from build123d import *

# Parameters (mm, degrees)
F0_W     = 30
F0_H     = 35
F0_H_2   = 5
F1_DEPTH = 4
F2_W     = 4.5
F2_H     = 40
F3_DEPTH = 7
F4_W     = 4.5
F4_H     = 40
F4_W_2   = 25.5
F5_DEPTH = 10
F7_D     = 6
F8_R     = 3
F9_DEPTH = 4.5
F10_SIZE = 8


# Not quite as in the source:
# - a feature names something its author has since deleted; it is built from what else it names


with BuildPart() as f1:
    # F0 (on Top) → F1 (new body)
    with BuildSketch(Plane.XY):
        with Locations((0, -22.5)):
            Rectangle(F0_W, F0_H)
        with Locations((0, -2.5)):
            Rectangle(F0_W, F0_H_2)
    extrude(amount=F1_DEPTH)

    # F2 (on face) → F3 (join)
    with BuildSketch(Plane.XY.offset(4)):
        with Locations((12.75, -20)):
            Rectangle(F2_W, F2_H)
        with Locations((-12.75, -20)):
            Rectangle(F2_W, F2_H)
    extrude(amount=F3_DEPTH)

    # F4 (on face) → F5 (join)
    with BuildSketch(Plane.XY.offset(11)):
        with Locations((12.75, -20)):
            Rectangle(F4_W, F4_H)
        with Locations((-2.25, -20)):
            Rectangle(F4_W_2, F4_H)
    extrude(amount=F5_DEPTH)

    # F7 (through all)
    with Locations(Plane.XY.offset(21)):
        with Locations((0, -20)):
            Hole(F7_D / 2)

    # F8 (on face) → F9 (cut)
    with BuildSketch(Plane(origin=(0, 0, 11), x_dir=(1, 0, 0), z_dir=(0, 0, -1))):
        Polygon((2.5980762114, 24.5), (-2.5980762114, 24.5), (-5.1961524227, 20), (-2.5980762114, 15.5), (2.5980762114, 15.5), (5.1961524227, 20), align=None)
        with Locations((0, 20)):
            Circle(F8_R, mode=Mode.SUBTRACT)
    extrude(amount=-F9_DEPTH, mode=Mode.SUBTRACT)

    # F10
    f10_edges = [f1.edges().sort_by_distance(p)[0] for p in [
        (-15, -20, 21),
        (15, -20, 21),
    ]]
    chamfer(f10_edges, length=F10_SIZE)


solid = f1.part
The model under review builds one solid part; all positions refer to its coordinate system, in mm. A direction names the side the tool comes from. Give positions to 0.01 mm unless a question says otherwise; leave off trailing zeros. Loops run counter-clockwise (first coordinate to the right, second up) from the corner with the lowest first, then second, coordinate; pieces in that order, holes last. Notation, with made-up numbers: (86.5, 58.25) -> (127.5, 58.25) arc R9 cw to (127.5, 64.25) -> close; hole circle Ø10 at (22, 62). An arc over 180 degrees is marked (long way). Answer as a JSON object with one key per item and string values. Group by question number.
Q1. Draft analysis for pull direction Z (two halves, no side actions). For faces 1 (the flat face through (0, -15.5, 13)), 2 (the flat face through (-4, -20, 0)), 3 (the flat face through (0, -40, 13)), state which applies: pulls with the +Z half, pulls with the -Z half, needs draft (parallel to the pull), parting line crosses it, or undercut.
Q2. Take a section at C-C (z = 12.25). Write out the cut boundary in (x, y).
Q3. Wall thickness on line 1 along Z through (x, y) = (-6.5, -22); line 2 along X through (y, z) = (-33, 9); line 3 along Y through (x, z) = (0, 16.95): over which ranges is each line inside the solid? List them lowest first.
Q4. Take a section at D-D (y = -16.5). Write out the cut boundary in (x, z), plus the area to 3 significant figures.
Q5. Take a section at A-A (x = 0). Write out the cut boundary in (y, z).
Q6. Insertion check: pin 1 (6 mm diameter, centred on x = 11, y = -10, fed in from +Z); pin 2 (2 mm diameter, centred on y = -31, z = 16, fed in from +X). Each pin has a flat end and moves straight along its axis. Give the tip position at first contact, or say it passes through.
Q7. Tool access review of faces 4 (the flat face through (-3.88, -22.28, 13.22)), 5 (the flat face through (-11, -20, 17)), 6 (the flat face through (-10.5, -20, 7)): name each direction out of +Z, -Z, +X, -X, +Y, -Y from which nothing blocks a thin tool from reaching the whole face with its end or side.
Q8. Take a section at B-B (z = 5.75). Write out the cut boundary in (x, y).
Answer below:
{
 "1": {"face 1": "undercut", "face 2": "pulls with the -Z half", "face 3": "needs draft"},
 "2": {"outline": "(-15, -40) -> (15, -40) -> (15, 0) -> (-15, 0) -> close; hole (-5.2, -20) -> (-2.6, -24.5) -> (2.6, -24.5) -> (5.2, -20) -> (2.6, -15.5) -> (-2.6, -15.5) -> close"},
 "3": {"line 1": "z = 0 to 4, 11 to 21", "line 2": "x = -15 to -10.5, 10.5 to 15", "line 3": "y = -40 to -23, -17 to 0"},
 "4": {"outline": "(-15, 0) -> (15, 0) -> (15, 13) -> (7, 21) -> (-7, 21) -> (-15, 13) -> close; hole (-10.5, 4) -> (10.5, 4) -> (10.5, 11) -> (3.18, 11) -> (3.18, 15.5) -> (-3.18, 15.5) -> (-3.18, 11) -> (-10.5, 11) -> close", "area": "390 mm2"},
 "5": {"outline": "(-40, 0) -> (-23, 0) -> (-23, 4) -> (-40, 4) -> close; (-40, 11) -> (-24.5, 11) -> (-24.5, 15.5) -> (-23, 15.5) -> (-23, 21) -> (-40, 21) -> close; (-17, 0) -> (0, 0) -> (0, 4) -> (-17, 4) -> close; (-17, 15.5) -> (-15.5, 15.5) -> (-15.5, 11) -> (0, 11) -> (0, 21) -> (-17, 21) -> close"},
 "6": {"pin 1": "stops at z = 20", "pin 2": "stops at x = 13"},
 "7": {"face 4": "none", "face 5": "+Z, -X, +Y, -Y", "face 6": "+Y, -Y"},
 "8": {"outline": "(-15, -40) -> (-10.5, -40) -> (-10.5, 0) -> (-15, 0) -> close; (10.5, -40) -> (15, -40) -> (15, 0) -> (10.5, 0) -> close"}
}
